Print and shaded views of the part. All mm, measured from the part's lowest x, y and z. Give positions to 0.01 mm unless a question says otherwise; leave off trailing zeros. Loops run counter-clockwise (first coordinate to the right, second up) from the corner with the lowest first, then second, coordinate; pieces in that order, holes last. Notation, with made-up numbers: M 79.25,37.5 L 135.25,37.5 A31 cw 135.25,67.5 Z; hole C 76,-20.75 d11. An arc over 180 degrees is marked long. Answer in a Markdown table with one row per item.
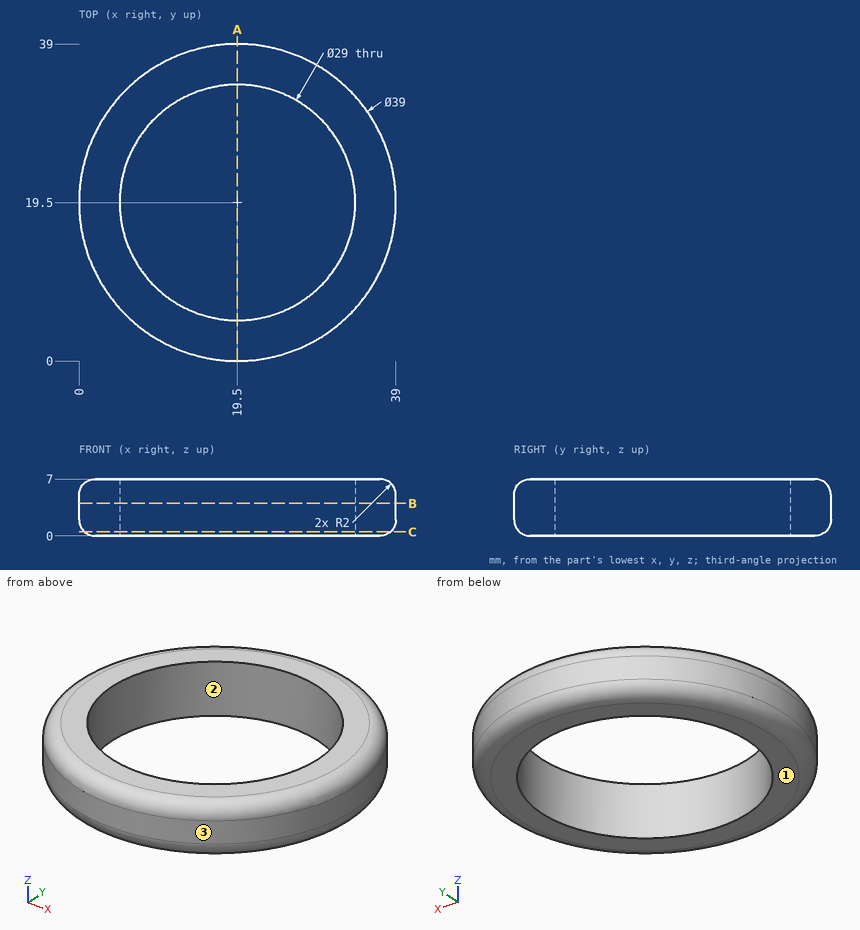
(1) Saw through at B-B, the plane z = 4. Give the cut face in (x, y), and give its area (3 significant figures).
Established:
| item | result |
|---|---|
| outline | C 19.5,19.5 d39; hole C 19.5,19.5 d29 |
| area | 534 mm2 |
(2) Mould opens along X. For the marked faces 1, 2 and 3 say: pulls with the +X half, pulls with the -X half, needs draft (parallel to the pull), parting line crosses it, or undercut.
Established:
| item | result |
|---|---|
| face 1 | needs draft |
| face 2 | undercut |
| face 3 | parting line crosses it |
(3) Wall check: L1, parallel to Y at x = 19.5, z = 2.5; L2, parallel to Y at x = 19.5, z = 5.5; L3, parallel to X at y = 27, z = 5.5. Give the ranges that are in metal, low to high.
Established:
| item | result |
|---|---|
| L1 | y = 0 to 5, 34 to 39 |
| L2 | y = 0.06 to 5, 34 to 38.94 |
| L3 | x = 1.57 to 7.09, 31.91 to 37.43 |
(4) Saw through at C-C, the plane z = 0.5. Give the cut face in (x, y).
Established:
| item | result |
|---|---|
| outline | C 19.5,19.5 d37.65; hole C 19.5,19.5 d29 |
(5) Saw through at A-A, the plane x = 19.5. Give the cut face in (y, z), and give its area (3 significant figures).
Established:
| item | result |
|---|---|
| outline | M 0,2 A2 ccw 2,0 L 5,0 L 5,7 L 2,7 A2 ccw 0,5 Z; M 34,0 L 37,0 A2 ccw 39,2 L 39,5 A2 ccw 37,7 L 34,7 Z |
| area | 66.6 mm2 |
(6) Flat gauge pins, fed straight in: P1, Ø4, axis at y = 16.5, z = 6.5, coming from the +X side; P2, Ø17.5, axis at x = 19.5, y = 19.5, coming from the -Z side. Where does each tip first touch, or does it go through?
Established:
| item | result |
|---|---|
| P1 | stops at x = 38.93 |
| P2 | passes through |
